```python
from build123d import *

# Parameters (mm, degrees)
SKETCH1_W           = 20
SKETCH1_H           = 20
BOSS_EXTRUDE1_DEPTH = 4
SKETCH2_R           = 3.7
CUT_EXTRUDE1_DEPTH  = 2.6
SKETCH3_R           = 2.1
CUT_EXTRUDE2_DEPTH  = 29.403520909
SKETCH4_W           = 12
SKETCH4_H           = 4
BOSS_EXTRUDE2_DEPTH = 12
SKETCH7_W           = 20
SKETCH7_H           = 4
BOSS_EXTRUDE3_DEPTH = 10
SKETCH8_W           = 8
SKETCH8_H           = 20
BOSS_EXTRUDE4_DEPTH = 5
SKETCH9_W           = 8
SKETCH9_H           = 20
BOSS_EXTRUDE5_DEPTH = 5
SKETCH10_R          = 1.6
CUT_EXTRUDE5_DEPTH  = 42.243181255
SKETCH11_W          = 30
SKETCH11_H          = 30
CUT_EXTRUDE6_DEPTH  = 6
SKETCH12_R          = 1.45
CUT_EXTRUDE7_DEPTH  = 42.243181255
SKETCH13_W          = 8
SKETCH13_H          = 20
BOSS_EXTRUDE6_DEPTH = 2
SKETCH14_W          = 8
SKETCH14_H          = 20
BOSS_EXTRUDE7_DEPTH = 2
SKETCH15_W          = 16
SKETCH15_H          = 12
CUT_EXTRUDE8_DEPTH  = 39.845849199
FILLET2_R           = 3
FILLET4_R           = 2
FILLET5_START       = -21
FILLET5_DEPTH       = 22
FILLET6_R           = 3
FILLET7_R           = 1
FILLET8_R           = 1


with BuildPart() as part:
    # Sketch1 → Boss-Extrude1 (new body)
    with BuildSketch(Plane(origin=(0, 0, 0), x_dir=(0, 0, -1), z_dir=(1, 0, 0))):
        with Locations((-10, -10)):
            Rectangle(SKETCH1_W, SKETCH1_H)
    extrude(amount=BOSS_EXTRUDE1_DEPTH)

    # Sketch2 → Cut-Extrude1 (cut)
    with BuildSketch(Plane(origin=(4, 0, 0), x_dir=(0, 0, -1), z_dir=(1, 0, 0))):
        with Locations((-10, -10)):
            Circle(SKETCH2_R)
    extrude(amount=-CUT_EXTRUDE1_DEPTH, mode=Mode.SUBTRACT)

    # Sketch3 → Cut-Extrude2 (cut, through all)
    with BuildSketch(Plane(origin=(1.4, 0, 0), x_dir=(0, 0, -1), z_dir=(1, 0, 0))):
        with Locations((-10, -10)):
            Circle(SKETCH3_R)
    extrude(amount=-CUT_EXTRUDE2_DEPTH, mode=Mode.SUBTRACT)

    # Sketch4 → Boss-Extrude2 (add)
    with BuildSketch(Plane(origin=(4, 0, 0), x_dir=(0, 0, -1), z_dir=(1, 0, 0))):
        Polygon((-20, 0), (-20, -20), (-16, -20), (-16, -16), (-16, -4), (-16, 0), align=None)
        with Locations((-10, -18)):
            Rectangle(SKETCH4_W, SKETCH4_H)
        Polygon((-4, -16), (-4, -20), (0, -20), (0, -4), (-4, -4), align=None)
        Polygon((0, 0), (-16, 0), (-16, -4), (-4, -4), (0, -4), align=None)
    extrude(amount=BOSS_EXTRUDE2_DEPTH)

    # Sketch7 → Boss-Extrude3 (add)
    with BuildSketch(Plane(origin=(16, 0, 0), x_dir=(0, 0, -1), z_dir=(1, 0, 0))):
        with Locations((-10, -18)):
            Rectangle(SKETCH7_W, SKETCH7_H)
        with Locations((-10, -2)):
            Rectangle(SKETCH7_W, SKETCH7_H)
    extrude(amount=BOSS_EXTRUDE3_DEPTH)

    # Sketch8 → Boss-Extrude4 (add)
    with BuildSketch(Plane(origin=(0, -20, 0), x_dir=(-1, 0, 0), z_dir=(0, -1, 0))):
        with Locations((-22, -10)):
            Rectangle(SKETCH8_W, SKETCH8_H)
    extrude(amount=BOSS_EXTRUDE4_DEPTH)

    # Sketch9 → Boss-Extrude5 (add)
    with BuildSketch(Plane(origin=(0, 0, 0), x_dir=(1, 0, 0), z_dir=(0, 1, 0))):
        with Locations((22, -10)):
            Rectangle(SKETCH9_W, SKETCH9_H)
    extrude(amount=BOSS_EXTRUDE5_DEPTH)

    # Sketch10 → Cut-Extrude5 (cut, through all)
    with BuildSketch(Plane(origin=(0, 0, 0), x_dir=(-1, 0, 0), z_dir=(0, 0, -1))):
        with Locations(Location((-22, 1, 0), (0, 0, 90))):
            Circle(SKETCH10_R)
        with Locations(Location((-22, -21, 0), (0, 0, 90))):
            Circle(SKETCH10_R)
    extrude(amount=-CUT_EXTRUDE5_DEPTH, mode=Mode.SUBTRACT)

    # Sketch11 → Cut-Extrude6 (cut)
    with BuildSketch(Plane.ZY):
        with Locations((15, -5)):
            Rectangle(SKETCH11_W, SKETCH11_H)
    extrude(amount=-CUT_EXTRUDE6_DEPTH, mode=Mode.SUBTRACT)

    # Sketch12 → Cut-Extrude7 (cut, through all)
    with BuildSketch(Plane(origin=(0, 0, 0), x_dir=(1, 0, 0), z_dir=(0, 1, 0))):
        with Locations(Location((11, -10, 0), (0, 0, 270))):
            Circle(SKETCH12_R)
    extrude(amount=-CUT_EXTRUDE7_DEPTH, mode=Mode.SUBTRACT)

    # Sketch13 → Boss-Extrude6 (add)
    with BuildSketch(Plane.XY.offset(20)):
        with Locations((10, -10)):
            Rectangle(SKETCH13_W, SKETCH13_H)
    extrude(amount=BOSS_EXTRUDE6_DEPTH)

    # Sketch14 → Boss-Extrude7 (add)
    with BuildSketch(Plane(origin=(0, 0, 0), x_dir=(-1, 0, 0), z_dir=(0, 0, -1))):
        with Locations((-10, -10)):
            Rectangle(SKETCH14_W, SKETCH14_H)
    extrude(amount=BOSS_EXTRUDE7_DEPTH)

    # Sketch15 → Cut-Extrude8 (cut, through all)
    with BuildSketch(Plane.ZY.offset(-6)):
        with Locations((10, -10)):
            Rectangle(SKETCH15_W, SKETCH15_H)
    extrude(amount=-CUT_EXTRUDE8_DEPTH, mode=Mode.SUBTRACT)

    # Fillet2
    fillet2_edges = [part.edges().sort_by_distance(p)[0] for p in [
        (26, -16, 10),
        (26, -4, 10),
    ]]
    fillet(fillet2_edges, radius=FILLET2_R)

    # Fillet4
    fillet4_edges = [part.edges().sort_by_distance(p)[0] for p in [
        (26, -25, 10),
        (18, -25, 10),
        (26, 5, 10),
        (18, 5, 10),
    ]]
    fillet(fillet4_edges, radius=FILLET4_R)

    # Fillet5: read off the stored shape, not the designer's step
    # Fillet5 outline → Fillet5 (cut)
    with BuildSketch(Plane(origin=(0, 0, 0), x_dir=(1, 0, 0), z_dir=(0, 1, 0)).offset(FILLET5_START)):
        with BuildLine():
            Line((6, 2), (6, -2))
            ThreePointArc((6, -2), (7.171572875, 0.828427125), (10, 2))
            Line((10, 2), (6, 2))
        make_face()
        with BuildLine():
            ThreePointArc((10, -22), (7.171572875, -20.828427125), (6, -18))
            Line((6, -18), (6, -22))
            Line((6, -22), (10, -22))
        make_face()
    extrude(amount=FILLET5_DEPTH, mode=Mode.SUBTRACT)

    # Fillet6
    # the kernel refuses this fillet: 3 mm, written as the material it takes off along each edge
    with BuildSketch(Plane(origin=(14, -27.071067812, -2), x_dir=(-1, 0, 0), z_dir=(0, 1, 0))) as fillet6_piece_1:
        with BuildLine():
            CenterArc((2.828427125, 3), FILLET6_R, 199.471220634, 70.528779366)
            Line((0, 2), (-0.056568542, 1.98))
            ThreePointArc((-0.056568542, 1.98), (-0.06, 1), (-0.06, 0))
            Line((-0.06, 0), (0, -0.06))
            Line((0, -0.06), (2.828427125, -0.06))
            Line((2.828427125, -0.06), (2.828427125, 0))
        make_face()
    extrude(amount=34.142135624, mode=Mode.SUBTRACT)
    with BuildSketch(Plane(origin=(14, -27.071067812, 22), x_dir=(0, 0, -1), z_dir=(0, 1, 0))) as fillet6_piece_2:
        with BuildLine():
            CenterArc((3, 2.828427125), FILLET6_R, 180, 70.528779366)
            Line((0, 2.828427125), (-0.06, 2.828427125))
            Line((-0.06, 2.828427125), (-0.06, 0))
            Line((-0.06, 0), (0, -0.06))
            ThreePointArc((0, -0.06), (1, -0.06), (1.98, -0.056568542))
            Line((1.98, -0.056568542), (2, 0))
        make_face()
    extrude(amount=34.142135624, mode=Mode.SUBTRACT)

    # Fillet7
    fillet7_edges = [part.edges().sort_by_distance(p)[0] for p in [
        (18, -20, 10),
    ]]
    fillet(fillet7_edges, radius=FILLET7_R)

    # Fillet8
    fillet8_edges = [part.edges().sort_by_distance(p)[0] for p in [
        (18, 0, 10),
    ]]
    fillet(fillet8_edges, radius=FILLET8_R)


solid = part.part
```
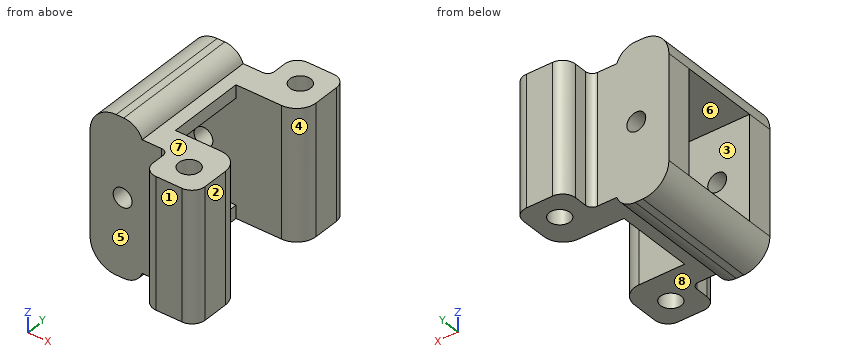
The model under review builds one solid part; all positions refer to its coordinate system, in mm. Face numbers are marked on the shaded views. A direction names the side the tool comes from. Round coordinates to 2 decimals unless told otherwise and drop trailing zeros. Order: outer loops, then holes, each group sorted by start corner. A loop starts at its lowest first (then second) coordinate and runs counter-clockwise, first axis right, second up. Notation, with made-up numbers: (9.5, -10) - (32.5, -10) arc R31 ccw to (32.5, 22) - close; hole circle Ø11 at (51, -27). An arc over 180 degrees is marked (long way). Answer in a Markdown table with one row per item.
(1) Take a section at C-C on y = -7. Write out the cut boundary in (x, z).
Result set:
| item | result |
|---|---|
| outline | (6, 2) arc R4 ccw to (10, -2) - (11.17, -2) arc R3 ccw to (14, 0) - (16, 0) - (16, 2) - close; (6, 18) - (16, 18) - (16, 20) - (14, 20) arc R3 ccw to (11.17, 22) - (10, 22) arc R4 ccw to start |
(2) Clearance check with flat-ended pins moving along their axes: P1, Ø1.6, axis at y = -8, z = 0.5, coming from the +X side; P2, Ø8.5, axis at x = 13.5, z = 8.5, coming from the +Y side; P3, Ø8.5, axis at x = 15.5, z = 7, coming from the -Y side. State where each tip first meets the part, or that it passes through.
Result set:
| item | result |
|---|---|
| P1 | stops at x = 16 |
| P2 | stops at y = 0.34 |
| P3 | stops at y = -24.98 |
(3) Mouldability with a two-part tool opening along Y and no side actions: class the marked faces 1, 2 and 3 as released by +Y, released by -Y, zero draft, split by the parting line, or undercut.
Result set:
| item | result |
|---|---|
| face 1 | released by -Y |
| face 2 | zero draft |
| face 3 | undercut |
(4) Machinability: for the marked faces 4, 5, 6, 7 and 8, which of the approach directions +Z, -Z, +X, -X, +Y, -Y give a long, thin tool a straight path to every point of the face, cutting with its end or side? Answer none if there is none.
Result set:
| item | result |
|---|---|
| face 4 | +Z, -Z, +X |
| face 5 | +Z, -Z, -X, -Y |
| face 6 | +X, -X |
| face 7 | +Z, +X, +Y, -Y |
| face 8 | -Z, +X, +Y, -Y |
(5) Take a section at D-D on x = 22. Write out the cut boundary in (y, z), plus the area to 3 significant figures.
Result set:
| item | result |
|---|---|
| outline | (-25, 0) - (-22.6, 0) - (-22.6, 20) - (-25, 20) - close; (-19.4, 0) - (-16, 0) - (-16, 20) - (-19.4, 20) - close; (-4, 0) - (-0.6, 0) - (-0.6, 20) - (-4, 20) - close; (2.6, 0) - (5, 0) - (5, 20) - (2.6, 20) - close |
| area | 232 mm2 |
(6) Take a section at B-B on z = 10. Count the separate pieces of the cut face and the enclosed holes in it, plus the area to 3 significant figures.
Result set:
| item | result |
|---|---|
| separate pieces | 4 |
| enclosed holes | 2 |
| area | 194 mm2 |
(7) For line 1 (X direction, y = -21, z = 15.75); line 2 (Y direction, x = 12.25, z = 11); line 3 (Y direction, x = 21, z = 6.25), list the stretches that pass through material, from the lowest coordinate up. Write a range as from..to.
Result set:
| item | result |
|---|---|
| line 1 | x = 18..20.4, 23.6..26 |
| line 2 | y = -20..-16, -4..0 |
| line 3 | y = -25..-22.25, -19.75..-16, -4..-0.25, 2.25..5 |
(8) Take a section at A-A on z = 15.5. Write out the cut boundary in (x, y), plus the area to 3 significant figures.
Result set:
| item | result |
|---|---|
| outline | (6, -20) - (17, -20) arc R1 cw to (18, -21) - (18, -23) arc R2 ccw to (20, -25) - (24, -25) arc R2 ccw to (26, -23) - (26, -19) arc R3 ccw to (23, -16) - (6, -16) - close; (6, -4) - (23, -4) arc R3 ccw to (26, -1) - (26, 3) arc R2 ccw to (24, 5) - (20, 5) arc R2 ccw to (18, 3) - (18, 1) arc R1 cw to (17, 0) - (6, 0) - close; hole circle Ø3.2 at (22, -21); hole circle Ø3.2 at (22, 1) |
| area | 217 mm2 |
